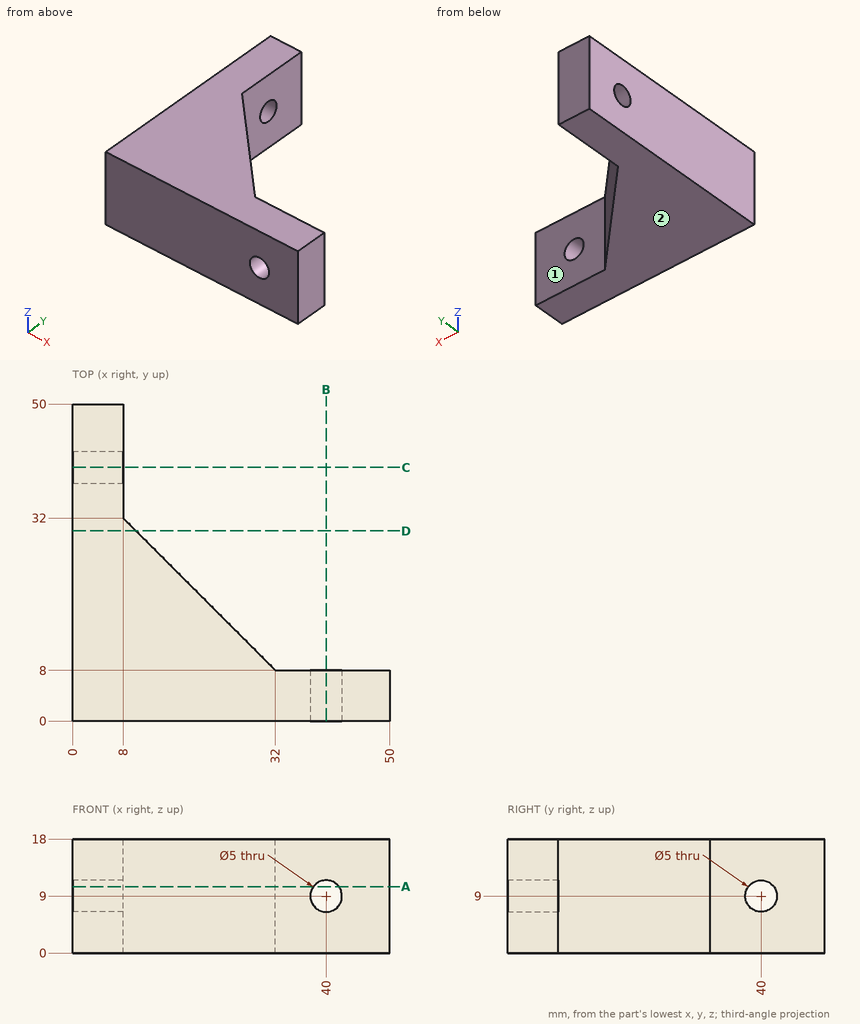
Here's the drawing with two shaded views (mm, measured from the low corner). I have some questions. A direction names the side the tool comes from. Round coordinates to 2 decimals unless told otherwise and drop trailing zeros. Loops run counter-clockwise (first coordinate to the right, second up) from the corner with the lowest first, then second, coordinate; pieces in that order, holes last. Notation, with made-up numbers: (-27.5, -6) -> (-1.5, -6) arc R16 cw to (-1.5, 21) -> close; hole circle Ø8 at (21.25, -13.5). An arc over 180 degrees is marked (long way). Answer as CSV lines item,"result". Start each with the question number.
1. I need wall thicknesses on probe 1 along Z at (x, y) = (1.75, 40); probe 2 along X at (y, z) = (2, 9); probe 3 along Y at (x, z) = (32, 7.25). Which ranges of each line are inside material? Lowest first, please. Write a range as from..to.
2. For the marked faces 1 and 2, which set-ups out of +Z, -Z, +X, -X, +Y, -Y let a thin tool reach every point of the face, with its end or its side?
3. Imagine slicing it at D-D on y = 30. Write out the boundary of the cut face in (x, z).
4. Imagine slicing it at B-B on x = 40. Write out the boundary of the cut face in (y, z).
5. I'm going to push flat-ended pins straight in: P1, Ø1.5, axis at y = 19, z = 15.5, coming from the +X side; P2, Ø9, axis at x = 42, z = 11, coming from the +Y side; P3, Ø3, axis at y = 21, z = 3, coming from the +X side. Where does each tip first touch, or does it pass through?
6. Imagine slicing it at A-A on z = 10.5. Write out the boundary of the cut face in (x, y).
Solution:
1,probe 1,"0..6.5, 11.5..18"
1,probe 2,"0..37.5, 42.5..50"
1,probe 3,"0..8"
2,face 1,"+Z, -Z, +X, +Y"
2,face 2,"-Z, +X, -X, +Y, -Y"
3,outline,"(0, 0) -> (10, 0) -> (10, 18) -> (0, 18) -> close"
4,outline,"(0, 0) -> (8, 0) -> (8, 6.5) -> (0, 6.5) -> close; (0, 11.5) -> (8, 11.5) -> (8, 18) -> (0, 18) -> close"
5,P1,"x = 21.75"
5,P2,"y = 8"
5,P3,"x = 20.5"
6,outline,"(0, 0) -> (38, 0) -> (38, 8) -> (32, 8) -> (8, 32) -> (8, 38) -> (0, 38) -> close; (0, 42) -> (8, 42) -> (8, 50) -> (0, 50) -> close; (42, 0) -> (50, 0) -> (50, 8) -> (42, 8) -> close"
